Could you check a few things on this drawing? It's one solid part, dimensions in mm from its lowest x, y, z. A direction names the side the tool comes from. Round coordinates to 2 decimals unless told otherwise and drop trailing zeros. Write each loop counter-clockwise with the first axis right and the second up, starting at its lowest first coordinate (ties: lowest second). Pieces come first, ordered by that corner, then holes. Notation, with made-up numbers: (89, 78) - (126, 78) arc R16 ccw to (126, 92) - close; hole circle Ø2 at (-27, 74). An arc over 180 degrees is marked (long way). Put each result on its own line as item: value.
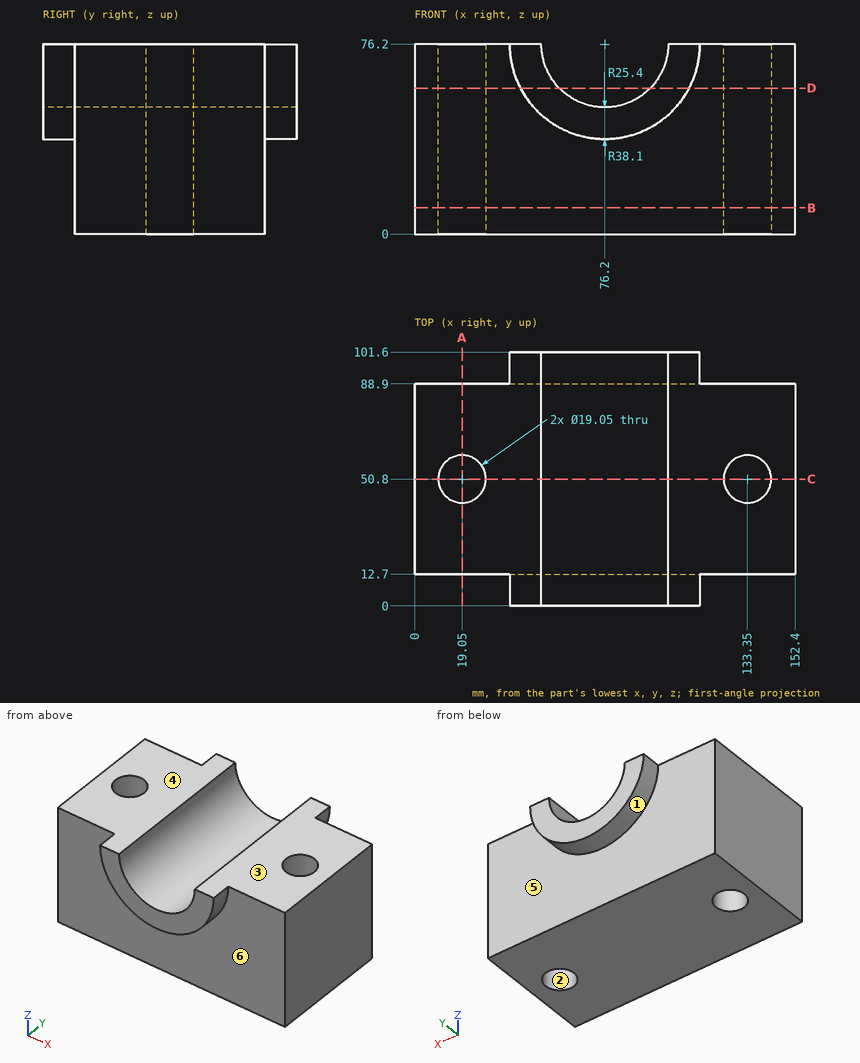
(1) Imagine slicing it at C-C, the plane y = 50.8. List the corners of the cut face in (x, z) for me (3 decimals), then the cut area to 3 significant figures.
Values found:
outline: (0, 0) - (9.525, 0) - (9.525, 76.2) - (0, 76.2) - close; (28.575, 0) - (123.825, 0) - (123.825, 76.2) - (101.6, 76.2) arc R25.4 cw to (50.8, 76.2) - (28.575, 76.2) - close; (142.875, 0) - (152.4, 0) - (152.4, 76.2) - (142.875, 76.2) - close
area: 7,700 mm^2
(2) Imagine slicing it at A-A, the plane x = 19.05. List the corners of the cut face in (y, z) for me (3 decimals), then the cut area to 3 significant figures.
Values found:
outline: (12.7, 0) - (41.275, 0) - (41.275, 76.2) - (12.7, 76.2) - close; (60.325, 0) - (88.9, 0) - (88.9, 76.2) - (60.325, 76.2) - close
area: 4,350 mm^2
(3) Imagine slicing it at D-D, the plane z = 58.5. List the corners of the cut face in (x, y) for me (3 decimals), then the cut area to 4 significant figures.
Values found:
outline: (0, 12.7) - (42.461, 12.7) - (42.461, 0) - (57.983, 0) - (57.983, 101.6) - (42.461, 101.6) - (42.461, 88.9) - (0, 88.9) - close; (94.417, 0) - (109.939, 0) - (109.939, 12.7) - (152.4, 12.7) - (152.4, 88.9) - (109.939, 88.9) - (109.939, 101.6) - (94.417, 101.6) - close; hole circle Ø19.05 at (19.05, 50.8); hole circle Ø19.05 at (133.35, 50.8)
area: 9,055 mm^2
(4) For the marked faces 4, 5 and 6, which set-ups out of +Z, -Z, +X, -X, +Y, -Y let a thin tool reach every point of the face, with its end or its side?
Values found:
face 4: +Z, +X, -X, +Y, -Y
face 5: -Z, +Y
face 6: -Z, -Y
(5) I'm going to push flat-ended pins straight in: pin 1 (12 mm diameter, centred on x = 122.5, z = 61.5, fed in from +Y); pin 2 (2 mm diameter, centred on x = 27.5, z = 17.5, fed in from -Y); pin 3 (25 mm diameter, centred on x = 19.05, y = 50.8, fed in from -Z). Where does each tip first touch, or does it pass through?
Values found:
pin 1: stops at y = 88.9
pin 2: stops at y = 12.7
pin 3: stops at z = 0
(6) Imagine slicing it at B-B, the plane z = 10.5. List the corners of the cut face in (x, y) for me (3 decimals).
Values found:
outline: (0, 12.7) - (152.4, 12.7) - (152.4, 88.9) - (0, 88.9) - close; hole circle Ø19.05 at (19.05, 50.8); hole circle Ø19.05 at (133.35, 50.8)
(7) Please list where these lines run through material, in increasing order: probe 1 along Y at (x, z) = (133.35, 39) (3 decimals); probe 2 along X at (y, z) = (50, 18); probe 3 along X at (y, z) = (45.5, 39). Write a range as from..to.
Values found:
probe 1: y = 12.7..41.275, 60.325..88.9
probe 2: x = 0..9.56, 28.54..123.86, 142.84..152.4
probe 3: x = 0..11.14, 26.96..125.44, 141.26..152.4
(8) If we mould it in two halves opening along X, with no side actions, what happens to the marked faces 1, 2 and 3? For each: pulls with the +X half, pulls with the -X half, needs draft (parallel to the pull), parting line crosses it, or undercut.
Values found:
face 1: parting line crosses it
face 2: undercut
face 3: needs draft
